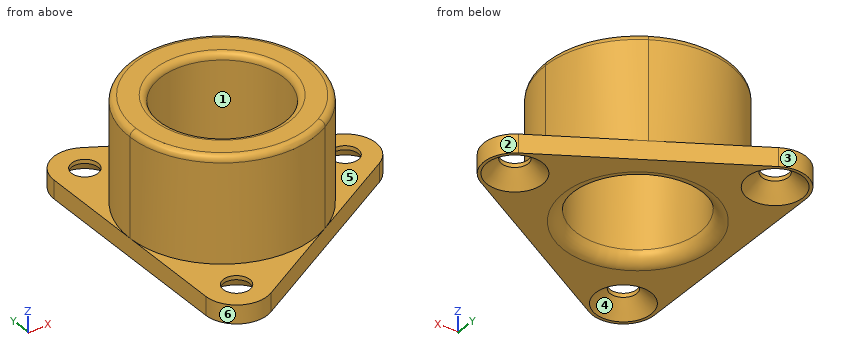
from build123d import *

# Parameters (mm, degrees)
F0_R           = 10
F1_DEPTH       = 20
F2_DEPTH       = 3
F3_D           = 4.3
F3_CSINK_D     = 9
F3_CSINK_ANGLE = 90
F4_R           = 2
F5_R           = 1


with BuildPart() as f1:
    # F0 (on Top) → F1 (new body)
    with BuildSketch(Plane.XY):
        with BuildLine():
            ThreePointArc((15, 0), (12.990381, 7.5), (7.5, 12.990381))
            ThreePointArc((7.5, 12.990381), (-7.5, 12.990381), (-15, 0))
            ThreePointArc((-15, 0), (-7.5, -12.990381), (7.5, -12.990381))
            ThreePointArc((7.5, -12.990381), (12.990381, -7.5), (15, 0))
        make_face()
        Circle(F0_R, mode=Mode.SUBTRACT)
    extrude(amount=F1_DEPTH)

    # F0 (on Top) → F2 (join)
    with BuildSketch(Plane.XY):
        with BuildLine():
            ThreePointArc((-15, 0), (-7.5, 12.990381), (7.5, 12.990381))
            Line((7.5, 12.990381), (-7.5, 21.650635))
            ThreePointArc((-7.5, 21.650635), (-12.5, 21.650635), (-15, 17.320508))
            Line((-15, 17.320508), (-15, 0))
        make_face()
        with BuildLine():
            ThreePointArc((22.5, -4.330127), (25, 0), (22.5, 4.330127))
            Line((22.5, 4.330127), (7.5, 12.990381))
            ThreePointArc((7.5, 12.990381), (12.990381, 7.5), (15, 0))
            ThreePointArc((15, 0), (12.990381, -7.5), (7.5, -12.990381))
            Line((7.5, -12.990381), (22.5, -4.330127))
        make_face()
        with BuildLine():
            ThreePointArc((7.5, -12.990381), (-7.5, -12.990381), (-15, 0))
            Line((-15, 0), (-15, -17.320508))
            ThreePointArc((-15, -17.320508), (-12.5, -21.650635), (-7.5, -21.650635))
            Line((-7.5, -21.650635), (7.5, -12.990381))
        make_face()
    extrude(amount=F2_DEPTH)

    # F3 (through all)
    with Locations(Plane(origin=(0, 0, 0), x_dir=(1, 0, 0), z_dir=(0, 0, -1))):
        with Locations((20, 0), (-10, -17.320508), (-10, 17.320508)):
            CounterSinkHole(F3_D / 2, F3_CSINK_D / 2, counter_sink_angle=F3_CSINK_ANGLE)

    # F4
    f4_edges = [f1.edges().sort_by_distance(p)[0] for p in [
        (-10, 0, 0),
    ]]
    fillet(f4_edges, radius=F4_R)

    # F5
    f5_edges = [f1.edges().sort_by_distance(p)[0] for p in [
        (-15, 0, 20),
        (-10, 0, 20),
    ]]
    fillet(f5_edges, radius=F5_R)


solid = f1.part
Could you check a few things on this model? Use its own coordinates, in mm. Face numbers are marked on the shaded views. A direction names the side the tool comes from. Give positions to 0.01 mm unless a question says otherwise; leave off trailing zeros. Loops run counter-clockwise (first coordinate to the right, second up) from the corner with the lowest first, then second, coordinate; pieces in that order, holes last. Notation, with made-up numbers: (75, 83.5) -> (97, 83.5) arc R22 cw to (97, 107.5) -> close; hole circle Ø2 at (3.25, 44.25). An arc over 180 degrees is marked (long way). Return JSON: item names as keys, results as strings.
Item 1: We'd pull the mould along Y, two halves only. Please class the marked faces 1, 2, 3 and 4: +Y half, -Y half, draft (parallel to the pull), parting line (faces both ways), or undercut.
Geometry results:
{"face 1": "undercut", "face 2": "parting line", "face 3": "+Y half", "face 4": "undercut"}
Item 2: I need wall thicknesses on L1, parallel to Y at x = 0, z = 11; L2, parallel to Z at x = 3, y = 15; L3, parallel to Y at x = 20, z = 2.75. Which ranges of each line are inside material? Lowest first, please. Write a range as from..to.
Geometry results:
{"L1": "y = -15..-10, 10..15", "L2": "z = 0..3", "L3": "y = -5.77..-2.15, 2.15..5.77"}
Item 3: If we section it at A-A on x = 20: List the corners of the cut face in (y, z) for me, plus the area to 3 significant figures.
Geometry results:
{"outline": "(-5.77, 0) -> (-4.5, 0) -> (-2.15, 2.35) -> (-2.15, 3) -> (-5.77, 3) -> close; (2.15, 2.35) -> (4.5, 0) -> (5.77, 0) -> (5.77, 3) -> (2.15, 3) -> close", "area": "16.2 mm²"}
Item 4: Which directions (+Z, -Z, +X, -X, +Y, -Y) give clear straight access to the entire face, cutting with the end or side of a thin tool? Please do the marked faces 5 and 6.
Geometry results:
{"face 5": "+Z, +X", "face 6": "+Z, -Z, -Y"}
Item 5: I'm going to push flat-ended pins straight in: pin 1 (3 mm diameter, centred on y = 14, z = 5, fed in from +X); pin 2 (12 mm diameter, centred on x = 1.5, z = 16.5, fed in from -Y); pin 3 (5 mm diameter, centred on y = -7, z = 4.5, fed in from -X); pin 4 (6 mm diameter, centred on y = 7, z = 12.5, fed in from +X). Where does each tip first touch, or does it pass through?
Geometry results:
{"pin 1": "stops at x = 8.29", "pin 2": "stops at y = -15", "pin 3": "stops at x = -15", "pin 4": "stops at x = 14.46"}
Item 6: If we section it at B-B on z = 7.5: List the corners of the cut face in (x, y) for me, plus the area to 3 significant figures.
Geometry results:
{"outline": "circle Ø30 at (0, 0); hole circle Ø20 at (0, 0)", "area": "393 mm²"}
